```python
from build123d import *

# Parameters (mm, degrees)
SKETCH1_W                = 14
SKETCH1_H                = 10
BOSS_EXTRUDE1_DEPTH      = 1
SKETCH2_W                = 5
SKETCH2_H                = 4
BOSS_EXTRUDE3_DEPTH      = 1
SKETCH3_W                = 5
SKETCH3_H                = 8.5
BOSS_EXTRUDE4_DEPTH      = 2
SKETCH4_R                = 0.5
CUT_EXTRUDE1_DEPTH       = 0.5
BOSS_EXTRUDE5_DEPTH      = 0.05
BOSS_EXTRUDE5_DEPTH_BACK = 1.05
SKETCH5_W                = 14
SKETCH5_H                = 0.75


with BuildPart() as part:
    # Sketch1 → Boss-Extrude1 (new body)
    with BuildSketch(Plane.XY):
        Rectangle(SKETCH1_W, SKETCH1_H)
    extrude(amount=BOSS_EXTRUDE1_DEPTH)

    # Sketch2 → Boss-Extrude3 (add)
    with BuildSketch(Plane.XY.offset(1)):
        Rectangle(SKETCH2_W, SKETCH2_H)
    extrude(amount=BOSS_EXTRUDE3_DEPTH)

    # Sketch3 → Boss-Extrude4 (add)
    with BuildSketch(Plane(origin=(0, 0, 0), x_dir=(-1, 0, 0), z_dir=(0, 0, -1))):
        with Locations((6, 0)):
            Rectangle(SKETCH3_W, SKETCH3_H)
        with Locations((-6, 0)):
            Rectangle(SKETCH3_W, SKETCH3_H)
    extrude(amount=BOSS_EXTRUDE4_DEPTH)

    # Sketch4 → Cut-Extrude1 (cut)
    with BuildSketch(Plane.XY.offset(2)):
        Circle(SKETCH4_R)
    extrude(amount=-CUT_EXTRUDE1_DEPTH, mode=Mode.SUBTRACT)

    # Sketch5 → Boss-Extrude5 (add, two sides: drawn at the far end of the back side and taken through both)
    with BuildSketch(Plane(origin=(0, 0, 0), x_dir=(-1, 0, 0), z_dir=(0, 0, -1)).offset(-BOSS_EXTRUDE5_DEPTH_BACK)):
        with Locations((0, 4.625)):
            Rectangle(SKETCH5_W, SKETCH5_H)
        with Locations((0, -4.625)):
            Rectangle(SKETCH5_W, SKETCH5_H)
    extrude(amount=BOSS_EXTRUDE5_DEPTH + BOSS_EXTRUDE5_DEPTH_BACK)


solid = part.part
```
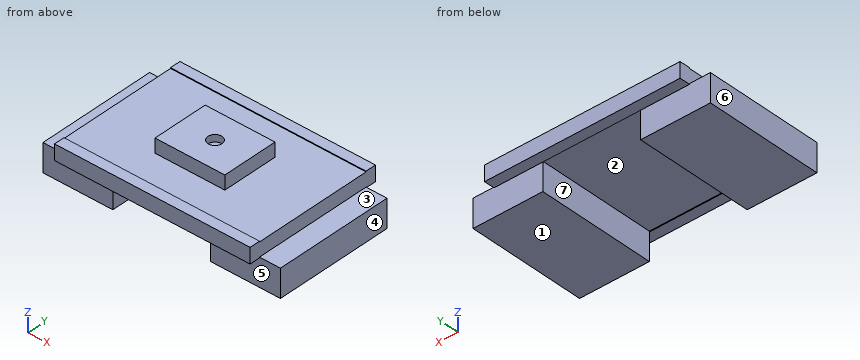
The model under review builds one solid part; all positions refer to its coordinate system, in mm. Face numbers are marked on the shaded views. A direction names the side the tool comes from. Round coordinates to 2 decimals unless told otherwise and drop trailing zeros. Loops run counter-clockwise (first coordinate to the right, second up) from the corner with the lowest first, then second, coordinate; pieces in that order, holes last.
Item 1: Clearance check with flat-ended pins moving along their axes: pin 1 Ø0.5 at (x, z) = (0, 1.5) entering from +Y; pin 2 Ø2 at (x, z) = (-4.5, -1.5) entering from +Y; pin 3 Ø1.6 at (x, z) = (-6, -1) entering from -Y. State where each tip first meets the part, or that it passes through.
Determined:
pin 1: stops at y = 2
pin 2: stops at y = 4.25
pin 3: stops at y = -4.25
Item 2: Take a section at C-C (z = -0.45). Write out the cut boundary in (x, y), then the cut area to 3 significant figures.
Determined:
outline: (-8.5, -4.25) - (-3.5, -4.25) - (-3.5, 4.25) - (-8.5, 4.25) - close; (3.5, -4.25) - (8.5, -4.25) - (8.5, 4.25) - (3.5, 4.25) - close
area: 85.0 mm2
Item 3: For the marked faces 1, 2 and 3, list the 3-axis set-ups (+Z, -Z, +X, -X, +Y, -Y) from which the entire face can be reached by the end or side of a thin tool; tool diameter is ignored.
Determined:
face 1: -Z, +X, -X, +Y, -Y
face 2: -Z
face 3: +Z, +X, +Y, -Y
Item 4: Take a section at D-D (y = 0). Write out the cut boundary in (x, z).
Determined:
outline: (-8.5, -2) - (-3.5, -2) - (-3.5, 0) - (3.5, 0) - (3.5, -2) - (8.5, -2) - (8.5, 0) - (7, 0) - (7, 1) - (2.5, 1) - (2.5, 2) - (0.5, 2) - (0.5, 1.5) - (-0.5, 1.5) - (-0.5, 2) - (-2.5, 2) - (-2.5, 1) - (-7, 1) - (-7, 0) - (-8.5, 0) - close
Item 5: For line 1 (X direction, y = -3.25, z = -1.5); line 2 (Y direction, x = 0, z = 1.6); line 3 (Z direction, x = -1.75, y = 1.75), list the stretches that pass through material, from the lowest coordinate up.
Determined:
line 1: x = -8.5 to -3.5, 3.5 to 8.5
line 2: y = -2 to -0.5, 0.5 to 2
line 3: z = 0 to 2
Item 6: Take a section at B-B (y = -2.25). Write out the cut boundary in (x, z), then the cut area to 3 significant figures.
Determined:
outline: (-8.5, -2) - (-3.5, -2) - (-3.5, 0) - (3.5, 0) - (3.5, -2) - (8.5, -2) - (8.5, 0) - (7, 0) - (7, 1) - (-7, 1) - (-7, 0) - (-8.5, 0) - close
area: 34.0 mm2
Item 7: Take a section at A-A (x = 5.5). Write out the cut boundary in (y, z), then the cut area to 4 significant figures.
Determined:
outline: (-5, -0.05) - (-4.25, -0.05) - (-4.25, -2) - (4.25, -2) - (4.25, -0.05) - (5, -0.05) - (5, 1.05) - (4.25, 1.05) - (4.25, 1) - (-4.25, 1) - (-4.25, 1.05) - (-5, 1.05) - close
area: 27.15 mm2
Item 8: Mouldability with a two-part tool opening along X and no side actions: class the marked faces 4, 5, 6 and 7 as released by +X, released by -X, zero draft, split by the parting line, or undercut.
Determined:
face 4: released by +X
face 5: zero draft
face 6: released by -X
face 7: undercut
